The listing builds one solid part. Answer for the finished solid, in the listing's coordinates (mm). Face numbers are marked on the shaded views. A direction names the side the tool comes from. Round coordinates to 2 decimals unless told otherwise and drop trailing zeros. Write each loop counter-clockwise with the first axis right and the second up, starting at its lowest first coordinate (ties: lowest second). Pieces come first, ordered by that corner, then holes.
Item 1: Find section B-B on x = 0. Give the vertices of the cut face in (y, z).
Item 2: A tool of negligible diameter and unlimited length cuts with its end or side. For the marked faces 4, 5, 6 and 7, from which of +Z, -Z, +X, -X, +Y, -Y can it reach the whole face along a straight path? Write none if from no direction.
Item 3: Find section C-C on y = 4.25. Give the vertices of the cut face in (x, z).
Item 4: Find the intervals of material crossed by probe 1 along Y at (x, z) = (0, 3.05); probe 2 along X at (y, z) = (0, 1.6); probe 3 along X at (y, z) = (0.5, 4.8), in increasing order.
Item 5: Each of these flat-tipped pins is pushed along its axis until it touches: pin 1 (3 mm diameter, centred on x = -1, z = 1.5, fed in from +Y); pin 2 (2 mm diameter, centred on x = 5.5, z = 2, fed in from +Y); pin 3 (1 mm diameter, centred on y = 5.5, z = 2, fed in from +X). Where does it stop, or does it pass through?
Item 6: Find section A-A on y = -0.25. Give the vertices of the cut face in (x, z), then the cut area to 3 significant figures.
Item 7: For a pull along X with two mould halves and no side action, classify the marked faces 1, 2 and 3 as +X half, -X half, draft (parallel to the pull), parting line (faces both ways), or undercut.
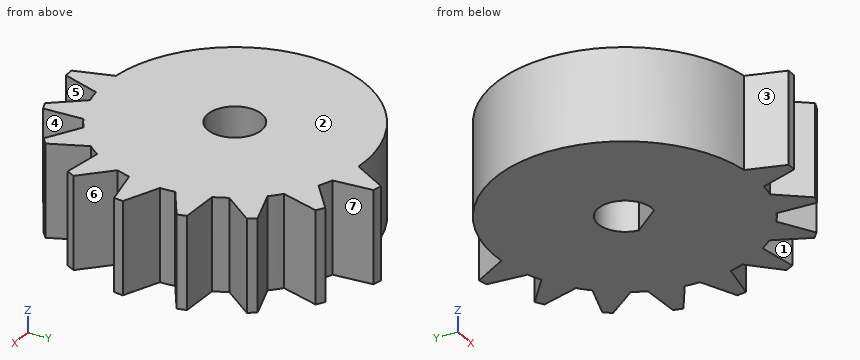
```python
from build123d import *

# Parameters (mm, degrees)
SKETCH1_R           = 7
BOSS_EXTRUDE1_DEPTH = 5
BOSS_EXTRUDE2_DEPTH = 5
CIRPATTERN3_COUNT   = 9
CIRPATTERN3_ANGLE   = 168
CUT_EXTRUDE1_START  = -3.5
SKETCH5_R           = 1.45
CUT_EXTRUDE1_DEPTH  = 3.5


with BuildPart() as part:
    # Sketch1 → Boss-Extrude1 (new body)
    with BuildSketch(Plane.XY):
        with Locations((0.027853283, 0.035186328)):
            Circle(SKETCH1_R)
        with BuildLine():
            Line((0.20260938, -1.435774857), (1.443945142, 0.132372307))
            ThreePointArc((1.443945142, 0.132372307), (-1.136906694, 0.899968427), (0.20260938, -1.435774857))
        make_face(mode=Mode.SUBTRACT)
    extrude(amount=BOSS_EXTRUDE1_DEPTH)

    # Sketch3 → Boss-Extrude2 (add)
    with BuildSketch(Plane(origin=(0, 0, 0), x_dir=(-1, 0, 0), z_dir=(0, 0, -1))):
        Polygon((0.857146717, -6.908643667), (-0.912853283, -6.908643667), (-0.277853283, -8.908643667), (0.222146717, -8.908643667), align=None)
    boss_extrude2 = extrude(amount=-BOSS_EXTRUDE2_DEPTH)

    # CirPattern3: Boss-Extrude2 ×9 about axis
    cirpattern3_axis = Axis((0.027853283, 0.035186328, 0), (0, 0, 1))
    for i in range(1, CIRPATTERN3_COUNT):
        add(boss_extrude2.rotate(cirpattern3_axis, i * CIRPATTERN3_ANGLE / (CIRPATTERN3_COUNT - 1)))

    # Sketch5 → Cut-Extrude1 (cut)
    with BuildSketch(Plane.XY.offset(5).offset(CUT_EXTRUDE1_START)):
        with Locations(Location((0, 0, 0), (0, 0, 278.032257946))):
            Circle(SKETCH5_R)
    extrude(amount=CUT_EXTRUDE1_DEPTH, mode=Mode.SUBTRACT)


solid = part.part
```
Check values:
1. outline: (-8.91, 0) - (-1.45, 0) - (-1.45, 5) - (-8.91, 5) - close; (1.45, 0) - (7.04, 0) - (7.04, 5) - (1.45, 5) - close
2. face 4: +Z, -Z
2. face 5: +Z, -Z, -Y
2. face 6: +Z, -Z, +X
2. face 7: +Z, -Z, +Y
3. outline: (-5.56, 0) - (6.79, 0) - (6.79, 5) - (-5.56, 5) - close
4. probe 1: y = -8.91 to -1.45, 1.45 to 7.04
4. probe 2: x = -6.97 to -1.45, 1.45 to 7.46
4. probe 3: x = -6.96 to -1.36, 1.36 to 7.01
5. pin 1: stops at y = 7.04
5. pin 2: stops at y = 7.67
5. pin 3: stops at x = 7.41
6. outline: (-6.97, 0) - (-1.43, 0) - (-1.43, 5) - (-6.97, 5) - close; (1.14, 0) - (8.03, 0) - (8.03, 5) - (1.43, 5) - (1.43, 1.5) - (1.14, 1.5) - close
6. area: 61.1 mm2
7. face 1: undercut
7. face 2: draft
7. face 3: -X half
